```python
from build123d import *

# Parameters (mm, degrees)
F0_W      = 155
F0_H      = 80.5
F1_DEPTH  = 9.5
F2_T      = -1.5
F3_W      = 155
F3_H      = 80.5
F3_W_2    = 152
F3_H_2    = 77.5
F3_W_3    = 150
F3_H_3    = 75.5
F4_DEPTH  = 1.5
F5_W      = 20
F5_H      = 8.7980394721
F6_DEPTH  = 2.501
F7_W      = 8.8
F7_H      = 4.4
F7_W_2    = 15.4
F7_H_2    = 7.7
F8_DEPTH  = 1.5
F9_R      = 2
F10_R     = 5
F11_R     = 3
F12_F1_R  = 4
F12_F2_R  = 4
F12_F3_R  = 4
F12_F4_R  = 4
F13_W     = 70.5
F13_H     = 9.5
F14_DEPTH = 2.7929007565
F15_W     = 70.5
F15_H     = 9.5
F16_DEPTH = 2.7929007565
F17_W     = 28
F17_H     = 9.5
F18_DEPTH = 2.501
F19_DEPTH = 1
F20_W     = 91.1511071026
F20_H     = 60.2068249136
F21_DEPTH = 22
F22_W     = 56.2
F22_H     = 20
F23_DEPTH = 91


with BuildPart() as f1:
    # F0 (on Top) → F1 (new body)
    with BuildSketch(Plane.XY):
        with Locations((77.5, 40.25)):
            Rectangle(F0_W, F0_H)
    extrude(amount=F1_DEPTH)

    # F2
    f2_openings = [f1.faces().sort_by_distance(p)[0] for p in [
        (77.5, 40.25, 9.5),
    ]]
    offset(amount=F2_T, openings=f2_openings)

    # F3 (on face) → F4 (join)
    with BuildSketch(Plane.XY.offset(9.5)):
        with Locations((77.5, 40.25)):
            Rectangle(F3_W, F3_H)
        with Locations((77.5, 40.25)):
            Rectangle(F3_W_2, F3_H_2, mode=Mode.SUBTRACT)
        with Locations((77.5, 40.25)):
            Rectangle(F3_W_2, F3_H_2)
        with Locations((77.5, 40.25)):
            Rectangle(F3_W_3, F3_H_3, mode=Mode.SUBTRACT)
    extrude(amount=F4_DEPTH)

    # F5 (on face) → F6 (cut, through all)
    with BuildSketch(Plane(origin=(0, 80.5, 0), x_dir=(-1, 0, 0), z_dir=(0, 1, 0))):
        with Locations((-48, 5.8990197361)):
            Rectangle(F5_W, F5_H)
    extrude(amount=-F6_DEPTH, mode=Mode.SUBTRACT)

    # F7 (on face) → F8 (cut, through all)
    with BuildSketch(Plane(origin=(0, 0, 0), x_dir=(1, 0, 0), z_dir=(0, 0, -1))):
        with Locations((23.3, -27.05)):
            Rectangle(F7_W, F7_H)
        with Locations((23.3, -22.65)):
            Rectangle(F7_W, F7_H)
        with Locations((23.3, -35.8)):
            Rectangle(F7_W_2, F7_H_2)
        with Locations((23.3, -43.5)):
            Rectangle(F7_W_2, F7_H_2)
        with Locations((23.3, -52.25)):
            Rectangle(F7_W, F7_H)
        with Locations((23.3, -56.65)):
            Rectangle(F7_W, F7_H)
    extrude(amount=-F8_DEPTH, mode=Mode.SUBTRACT)

    # F9
    f9_edges = [f1.edges().sort_by_distance(p)[0] for p in [
        (18.9, 29.25, 0.75),
        (15.6, 47.35, 0.75),
        (18.9, 58.85, 0.75),
        (18.9, 20.45, 0.75),
        (15.6, 31.95, 0.75),
        (27.7, 50.05, 0.75),
        (31, 31.95, 0.75),
        (27.7, 20.45, 0.75),
        (27.7, 29.25, 0.75),
        (31, 47.35, 0.75),
        (27.7, 58.85, 0.75),
        (58, 79.75, 1.5),
        (38, 79.75, 1.5),
    ]]
    fillet(f9_edges, radius=F9_R)

    # F10
    f10_edges = [f1.edges().sort_by_distance(p)[0] for p in [
        (0, 0, 5.5),
        (0, 80.5, 5.5),
        (155, 0, 5.5),
        (155, 80.5, 5.5),
    ]]
    fillet(f10_edges, radius=F10_R)

    # F11
    f11_edges = [f1.edges().sort_by_distance(p)[0] for p in [
        (1.5, 79, 5.5),
        (1.5, 1.5, 5.5),
        (153.5, 79, 5.5),
        (153.5, 1.5, 5.5),
    ]]
    fillet(f11_edges, radius=F11_R)

    # F12: fillet of radius 4 on 4 edges, made by hand

    # F12_f1
    f12_f1_edges = [f1.edges().sort_by_distance(p)[0] for p in [
        (152.5, 78, 10.25),
    ]]
    fillet(f12_f1_edges, radius=F12_F1_R)

    # F12_f2
    f12_f2_edges = [f1.edges().sort_by_distance(p)[0] for p in [
        (2.5, 78, 10.25),
    ]]
    fillet(f12_f2_edges, radius=F12_F2_R)

    # F12_f3
    f12_f3_edges = [f1.edges().sort_by_distance(p)[0] for p in [
        (152.5, 2.5, 10.25),
    ]]
    fillet(f12_f3_edges, radius=F12_F3_R)

    # F12_f4
    f12_f4_edges = [f1.edges().sort_by_distance(p)[0] for p in [
        (2.5, 2.5, 10.25),
    ]]
    fillet(f12_f4_edges, radius=F12_F4_R)

    # F13 (on face) → F14 (cut, through all)
    with BuildSketch(Plane(origin=(0, 0, 0), x_dir=(0, -1, 0), z_dir=(-1, 0, 0))):
        with Locations((-40.25, 6.25)):
            Rectangle(F13_W, F13_H)
    extrude(amount=-F14_DEPTH, mode=Mode.SUBTRACT)

    # F15 (on face) → F16 (cut, through all)
    with BuildSketch(Plane.YZ.offset(155)):
        with Locations((40.25, 6.25)):
            Rectangle(F15_W, F15_H)
    extrude(amount=-F16_DEPTH, mode=Mode.SUBTRACT)

    # F17 (on face) → F18 (cut, through all)
    with BuildSketch(Plane.XZ):
        with Locations((37.5, 6.25)):
            Rectangle(F17_W, F17_H)
    extrude(amount=-F18_DEPTH, mode=Mode.SUBTRACT)

    # F19 (add): a face of the model
    f19_faces = [f1.faces().sort_by_distance(p)[0] for p in [
        (79.0729751372, 40.2079373473, 1.5),
    ]]
    extrude(f19_faces, amount=F19_DEPTH)

    # F20 (on face) → F21 (join)
    with BuildSketch(Plane(origin=(0, 0, 0), x_dir=(1, 0, 0), z_dir=(0, 0, -1))):
        with Locations((98.8614168018, -39.4122553989)):
            Rectangle(F20_W, F20_H)
    extrude(amount=F21_DEPTH)

    # F22 (on face) → F23 (cut)
    with BuildSketch(Plane(origin=(53.2858632505, 0, 0), x_dir=(0, -1, 0), z_dir=(-1, 0, 0))):
        with Locations((-39.4156678557, -10)):
            Rectangle(F22_W, F22_H)
    extrude(amount=-F23_DEPTH, mode=Mode.SUBTRACT)


solid = f1.part
```
Here's how the part is built. I have some questions about the finished solid (model axes, mm). A direction names the side the tool comes from. Coordinates: 2 decimals unless noted, no trailing zeros. Order: outer loops, then holes, each group sorted by start corner. A loop starts at its lowest first (then second) coordinate and runs counter-clockwise, first axis right, second up.
1) Imagine slicing it at C-C on x = 61. List the corners of the cut face in (y, z) for me.
2) Imagine slicing it at A-A on y = 41. List the corners of the cut face in (x, z) for me, and give its area (3 significant figures).
3) Which directions (+Z, -Z, +X, -X, +Y, -Y) give clear straight access to the entire face, cutting with the end or side of a thin tool? Please do faces 1 (the face through (98, 69.516, -11)), 2 (the face through (154, 75.5, 8)), 3 (the face through (10, 2, 9.5)), 4 (the face through (98, 9.309, -11)).
4) Imagine slicing it at B-B on z = 8. List the corners of the cut face in (x, y) for me.
5) Imagine slicing it at D-D on y = 17.5. List the corners of the cut face in (x, z) for me.
6) I need wall thicknesses on line 1 (Y direction, x = 138.5, z = 4.5); line 2 (Y direction, x = 111, z = -12.5); line 3 (Z direction, x = 63.5, y = 57.5). Which ranges of each line are inside material? Lowest first, please.
7) Will these pins go through, and if not, where does the flat tip stop? pin 1 (16 mm diameter, centred on x = 115.5, z = -12, fed in from +Y); pin 2 (3 mm diameter, centred on y = 79, z = 7.5, fed in from +X); pin 3 (3 mm diameter, centred on x = 11, y = 3.5, fed in from -Z).
8) We'd pull the mould along Y, two halves only. Please class faces 5 (the face through (154, 5, 8)), 6 (the face through (14, 1.5, 6)), 7 (the face through (2, 1, 6)), 8 (the face through (144.437, 40, -11)): +Y half, -Y half, draft (parallel to the pull), parting line (faces both ways), or undercut.
Response values:
1. outline: (0, 0) - (9.31, 0) - (9.31, -22) - (69.52, -22) - (69.52, 0) - (80.5, 0) - (80.5, 11) - (78, 11) - (78, 9.5) - (79, 9.5) - (79, 2.5) - (1.5, 2.5) - (1.5, 9.5) - (2.5, 9.5) - (2.5, 11) - (0, 11) - close; hole (11.32, -20) - (67.52, -20) - (67.52, 0) - (11.32, 0) - close
2. outline: (0, 0) - (15.6, 0) - (15.6, 2.5) - (0, 2.5) - close; (31, 0) - (144.29, 0) - (144.29, -20) - (53.29, -20) - (53.29, -22) - (144.44, -22) - (144.44, 0) - (155, 0) - (155, 2.5) - (31, 2.5) - close
2. area: 534 mm2
3. face 1: -Z, +X, -X, +Y
3. face 2: +Z, +X, -X
3. face 3: none
3. face 4: -Z, +X, -X, -Y
4. outline: (0, 5) arc R5 ccw to (5, 0) - (23.5, 0) - (23.5, 1.5) - (4.5, 1.5) arc R3 cw to (1.5, 4.5) - (1.5, 5) - close; (0, 75.5) - (1.5, 75.5) - (1.5, 76) arc R3 cw to (4.5, 79) - (38, 79) - (38, 80.5) - (5, 80.5) arc R5 ccw to start; (51.5, 0) - (150, 0) arc R5 ccw to (155, 5) - (153.5, 5) - (153.5, 4.5) arc R3 cw to (150.5, 1.5) - (51.5, 1.5) - close; (58, 79) - (150.5, 79) arc R3 cw to (153.5, 76) - (153.5, 75.5) - (155, 75.5) arc R5 ccw to (150, 80.5) - (58, 80.5) - close
5. outline: (0, 0) - (144.29, 0) - (144.29, -20) - (53.29, -20) - (53.29, -22) - (144.44, -22) - (144.44, 0) - (155, 0) - (155, 2.5) - (0, 2.5) - close
6. line 1: y = 0 to 1.5, 79 to 80.5
6. line 2: y = 9.31 to 11.32, 67.52 to 69.52
6. line 3: z = -22 to -20, 0 to 2.5
7. pin 1: stops at y = 69.52
7. pin 2: stops at x = 154.58
7. pin 3: stops at z = 0
8. face 5: undercut
8. face 6: undercut
8. face 7: -Y half
8. face 8: draft
